CAD build for the part. Positions are in the model's coordinates, mm. Coordinates: 2 decimals unless noted, no trailing zeros. Write each loop counter-clockwise with the first axis right and the second up, starting at its lowest first coordinate (ties: lowest second). Pieces come first, ordered by that corner, then holes.
```python
from build123d import *

# Parameters (mm, degrees)
F1_DEPTH = 25.4


with BuildPart() as f1:
    # F0 (on Front) → F1 (new body)
    with BuildSketch(Plane.XZ):
        with BuildLine():
            Line((127, 190.5), (127, 178.223333))
            Line((127, 178.223333), (0, 178.223333))
            ThreePointArc((0, 178.223333), (-178.223333, 0), (0, -178.223333))
            Line((0, -178.223333), (127, -178.223333))
            Line((127, -178.223333), (127, -190.5))
            Line((127, -190.5), (190.5, -190.5))
            Line((190.5, -190.5), (190.5, -178.223333))
            Line((190.5, -178.223333), (190.5, -127))
            Line((190.5, -127), (127, -127))
            Line((127, -127), (0, -127))
            ThreePointArc((0, -127), (-127, 0), (0, 127))
            Line((0, 127), (127, 127))
            Line((127, 127), (190.5, 127))
            Line((190.5, 127), (190.5, 178.223333))
            Line((190.5, 178.223333), (190.5, 190.5))
            Line((190.5, 190.5), (127, 190.5))
        make_face()
    extrude(amount=F1_DEPTH)


solid = f1.part
```
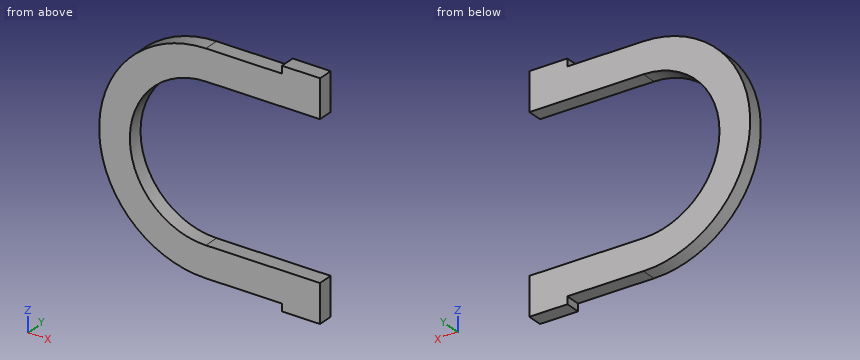
Item 1: Wall check: line 1 along Z through (x, y) = (61, -22.25); line 2 along Z through (x, y) = (160.5, -18); line 3 along X through (y, z) = (-8.75, -3.5). Give the ranges that are in metal, low to high.
Item 2: Flat gauge pins, fed straight in: pin 1 Ø12 at (x, y) = (-88.5, -8.5) entering from +Z; pin 2 Ø4 at (y, z) = (-21, 49) entering from +X; pin 3 Ø6 at (y, z) = (-19.5, 38.5) entering from -X. Where does each tip first touch, or does it go through?
Item 3: Saw through at B-B, the plane y = -11. Write the cut outline in (x, z), and give its area (3 significant figures).
Item 4: Saw through at A-A, the plane x = 15.5. Write the cut outline in (y, z), and give its area (3 significant figures).
Item 5: Saw through at C-C, the plane z = 0. Write the cut outline in (x, y).
Item 6: Saw through at D-D, the plane x = -55.5. Write the cut outline in (y, z), and give its area (3 significant figures).
Working result:
1. line 1: z = -178.22 to -127, 127 to 178.22
1. line 2: z = -190.5 to -127, 127 to 190.5
1. line 3: x = -178.19 to -126.95
2. pin 1: stops at z = 157.98
2. pin 2: stops at x = -116.31
2. pin 3: stops at x = -174.65
3. outline: (0, -178.22) - (127, -178.22) - (127, -190.5) - (190.5, -190.5) - (190.5, -127) - (0, -127) arc R127 cw to (0, 127) - (190.5, 127) - (190.5, 190.5) - (127, 190.5) - (127, 178.22) - (0, 178.22) arc R178.22 ccw to start
3. area: 45,600 mm2
4. outline: (-25.4, -178.22) - (0, -178.22) - (0, -127) - (-25.4, -127) - close; (-25.4, 127) - (0, 127) - (0, 178.22) - (-25.4, 178.22) - close
4. area: 2,600 mm2
5. outline: (-178.22, -25.4) - (-127, -25.4) - (-127, 0) - (-178.22, 0) - close
6. outline: (-25.4, -169.36) - (0, -169.36) - (0, -114.23) - (-25.4, -114.23) - close; (-25.4, 114.23) - (0, 114.23) - (0, 169.36) - (-25.4, 169.36) - close
6. area: 2,800 mm2
